from build123d import *

# Parameters (mm, degrees)
SKETCH_1_W          = 172.6
SKETCH_1_H          = 78
SKETCH_1_R          = 1.25
EXTRUDE_1_DEPTH     = 5
SKETCH_2_W          = 21.3
SKETCH_2_H          = 44
CUT_EXTRUDE_1_DEPTH = 95.835067354
SKETCH_1_3_R        = 2
CUT_EXTRUDE_2_DEPTH = 3.5
SKETCH_3_R          = 0.9
CUT_EXTRUDE_3_DEPTH = 95.835067354
SKETCH_4_R          = 15
CUT_EXTRUDE_4_DEPTH = 95.835067354
SKETCH_5_R          = 0.75
CUT_EXTRUDE_5_DEPTH = 95.835067354


with BuildPart() as part:
    # 草图1 → 凸台-拉伸1 (new body)
    with BuildSketch(Plane(origin=(0, 0, 0), x_dir=(1, 0, 0), z_dir=(0, 1, 0))):
        Rectangle(SKETCH_1_W, SKETCH_1_H)
        with Locations(Location((-73.15, 30.5, 0), (0, 0, 270))):
            Circle(SKETCH_1_R, mode=Mode.SUBTRACT)
        with Locations(Location((-73.15, -30.5, 0), (0, 0, 270))):
            Circle(SKETCH_1_R, mode=Mode.SUBTRACT)
        with Locations(Location((73.15, 30.5, 0), (0, 0, 270))):
            Circle(SKETCH_1_R, mode=Mode.SUBTRACT)
        with Locations(Location((73.15, -30.5, 0), (0, 0, 270))):
            Circle(SKETCH_1_R, mode=Mode.SUBTRACT)
    extrude(amount=EXTRUDE_1_DEPTH)

    # 草图2 → 切除-拉伸1 (cut, through all)
    with BuildSketch(Plane(origin=(0, 5, 0), x_dir=(1, 0, 0), z_dir=(0, 1, 0))):
        with Locations((-75.65, 0)):
            Rectangle(SKETCH_2_W, SKETCH_2_H)
        with Locations((75.65, 0)):
            Rectangle(SKETCH_2_W, SKETCH_2_H)
    extrude(amount=-CUT_EXTRUDE_1_DEPTH, mode=Mode.SUBTRACT)

    # 草图1<3> → 切除-拉伸2 (cut)
    with BuildSketch(Plane(origin=(0, 0, 0), x_dir=(1, 0, 0), z_dir=(0, 1, 0))):
        with Locations(Location((-73.15, 30.5, 0), (0, 0, 90))):
            Circle(SKETCH_1_3_R)
        with Locations(Location((-73.15, -30.5, 0), (0, 0, 90))):
            Circle(SKETCH_1_3_R)
        with Locations(Location((73.15, 30.5, 0), (0, 0, 90))):
            Circle(SKETCH_1_3_R)
        with Locations(Location((73.15, -30.5, 0), (0, 0, 90))):
            Circle(SKETCH_1_3_R)
    extrude(amount=CUT_EXTRUDE_2_DEPTH, mode=Mode.SUBTRACT)

    # 草图3 → 切除-拉伸3 (cut, through all)
    with BuildSketch(Plane(origin=(0, 5, 0), x_dir=(1, 0, 0), z_dir=(0, 1, 0))):
        with Locations(Location((-35, 35, 0), (0, 0, 270))):
            Circle(SKETCH_3_R)
        with Locations(Location((35, 35, 0), (0, 0, 270))):
            Circle(SKETCH_3_R)
        with Locations(Location((-35, -35, 0), (0, 0, 270))):
            Circle(SKETCH_3_R)
        with Locations(Location((35, -35, 0), (0, 0, 270))):
            Circle(SKETCH_3_R)
    extrude(amount=-CUT_EXTRUDE_3_DEPTH, mode=Mode.SUBTRACT)

    # 草图4 → 切除-拉伸4 (cut, through all)
    with BuildSketch(Plane.XZ):
        with Locations(Location((0, 0, 0), (0, 0, 270))):
            Circle(SKETCH_4_R)
    extrude(amount=-CUT_EXTRUDE_4_DEPTH, mode=Mode.SUBTRACT)

    # 草图5 → 切除-拉伸5 (cut, through all)
    with BuildSketch(Plane(origin=(0, 5, 0), x_dir=(1, 0, 0), z_dir=(0, 1, 0))):
        with Locations(Location((0, 21, 0), (0, 0, 270))):
            Circle(SKETCH_5_R)
        with Locations(Location((21, 0, 0), (0, 0, 270))):
            Circle(SKETCH_5_R)
        with Locations(Location((-21, 0, 0), (0, 0, 270))):
            Circle(SKETCH_5_R)
        with Locations(Location((0, -21, 0), (0, 0, 270))):
            Circle(SKETCH_5_R)
    extrude(amount=-CUT_EXTRUDE_5_DEPTH, mode=Mode.SUBTRACT)


solid = part.part
CAD build for the part. Positions are in the model's coordinates, mm. A direction names the side the tool comes from. Round coordinates to 2 decimals unless told otherwise and drop trailing zeros. Write each loop counter-clockwise with the first axis right and the second up, starting at its lowest first coordinate (ties: lowest second). Pieces come first, ordered by that corner, then holes. Notation, with made-up numbers: M 31.5,-21 L 64.5,-21 A15 ccw 64.5,-2 Z; hole C 60,57 d4. An arc over 180 degrees is marked long. Use a Markdown table: item, result. Add a question column.
1. Pull direction X, two halves, no side cores. Call faces 5 (the face through (-65, 3, 0)), 6 (the face through (76, 3, -22)), 7 (the face through (73, 3.5, 29)): released by +X, released by -X, zero draft, split by the parting line, or undercut.
2. Slice it at C-C on z = 3. Give the cut face in (x, y).
3. Slice it at A-A on y = 1.85. Give the number of separate pieces and of enclosed holes in the cut face, then the cut area to 3 significant figures.
4. Drill centre lines: probe 1 along Z at (x, y) = (73.5, 0.4); probe 2 along Z at (x, y) = (73.15, 4.2); probe 3 along X at (y, z) = (1.1, -30.5). Where is each one in solid material? Low to high.
5. Flat gauge pins, fed straight in: P1, Ø1.2, axis at x = -73.5, z = -30, coming from the -Y side; P2, Ø2, axis at y = 4.5, z = -16.5, coming from the +X side. Where does each tip first touch, or does it go through?
6. 3-axis set-ups, long thin cutter, end or side, ignore diameter. For faces 1 (the face through (-71.376, 1.726, 29.577)), 2 (the face through (-1, 0, -18)), 3 (the face through (76, 3, 22)), 4 (the face through (-76, 3, -22)): which of +Z, -Z, +X, -X, +Y, -Y reach the whole face in a straight line?
7. Slice it at B-B on x = 69. Give the cut face in (y, z), then the cut area to 3 significant figures.
Reply:
| question | item | result |
|---|---|---|
| 1 | face 5 | released by -X |
| 1 | face 6 | zero draft |
| 1 | face 7 | undercut |
| 2 | outline | M -65,0 L -14.7,0 L -14.7,5 L -65,5 Z; M 14.7,0 L 65,0 L 65,5 L 14.7,5 Z |
| 3 | separate pieces | 1 |
| 3 | enclosed holes | 13 |
| 3 | area | 10,800 mm^2 |
| 4 | probe 1 | z = -39 to -32.47, -28.53 to -22, 22 to 28.53, 32.47 to 39 |
| 4 | probe 2 | z = -39 to -31.75, -29.25 to -22, 22 to 29.25, 31.75 to 39 |
| 4 | probe 3 | x = -86.3 to -75.15, -71.15 to 71.15, 75.15 to 86.3 |
| 5 | P1 | passes through |
| 5 | P2 | stops at x = 65 |
| 6 | face 1 | -Y |
| 6 | face 2 | +Z, -Z, +X, -X, -Y |
| 6 | face 3 | +X, +Y, -Y |
| 6 | face 4 | -X, +Y, -Y |
| 7 | outline | M 0,-39 L 5,-39 L 5,-22 L 0,-22 Z; M 0,22 L 5,22 L 5,39 L 0,39 Z |
| 7 | area | 170 mm^2 |
